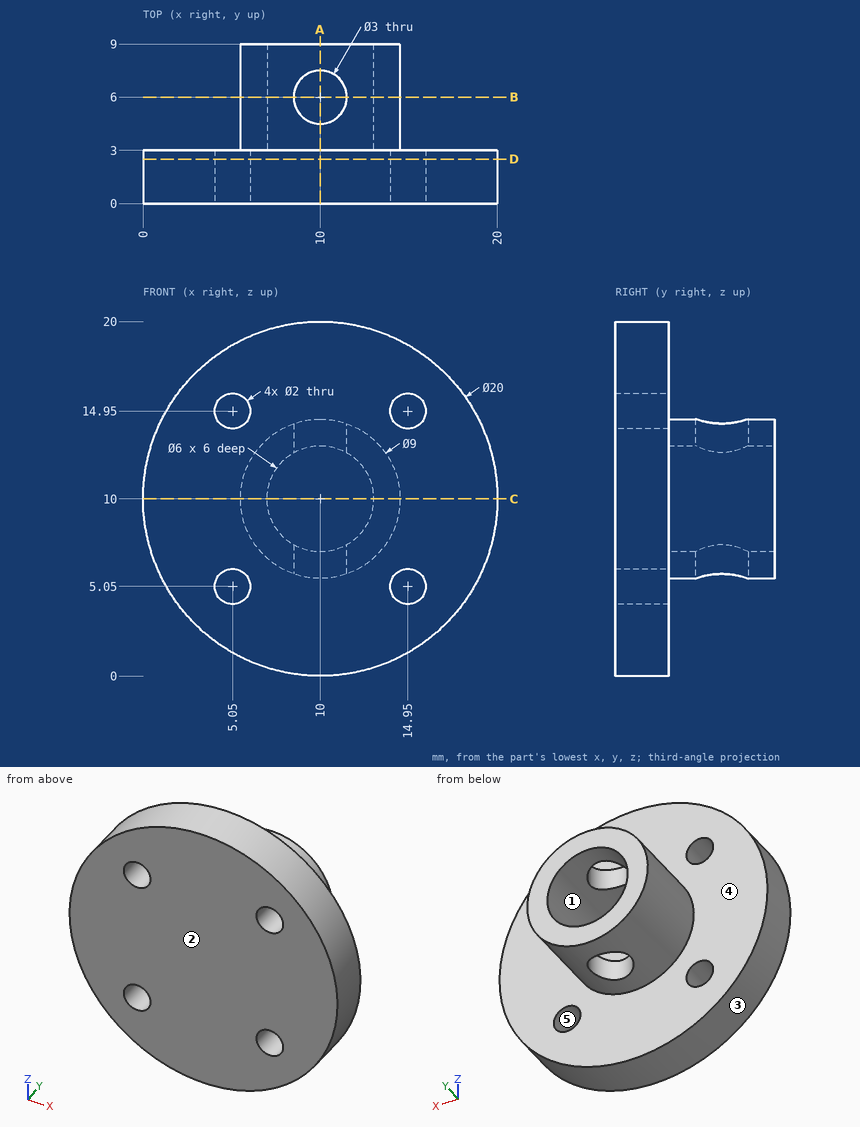
Answer from the drawing. Dimensions are ordinates in mm from the lowest x, y and z of the part. A direction names the side the tool comes from. Round coordinates to 2 decimals unless told otherwise and drop trailing zeros. Loops run counter-clockwise (first coordinate to the right, second up) from the corner with the lowest first, then second, coordinate; pieces in that order, holes last.
1) For the marked faces 1 and 2, determine the directions among +Z, -Z, +X, -X, +Y, -Y from which every point of the face is accessible in a straight line to the end or side of a thin tool.
Outcome:
face 1: +Y
face 2: +Z, -Z, +X, -X, -Y
2) Given P1, Ø5.5, axis at x = 10, z = 10, coming from the -Y side; P2, Ø4, axis at x = 10, y = 8, coming from the -Z side; P3, Ø2, axis at x = 15.5, y = 1.5, coming from the -Z side; P4, Ø1.5, axis at x = 12, y = 8, coming from the -Z side, each flat-ended and moving along its own axis, determine where each tip first touches the part or whether it passes through.
Outcome:
P1: stops at y = 0
P2: stops at z = 5.5
P3: stops at z = 1.07
P4: stops at z = 5.68
3) Consider line 1 (X direction, y = 5.25, z = 10); line 2 (Y direction, x = 5.5, z = 18); line 3 (Z direction, x = 15, y = 2.75). Determine where each line is inside the solid, lowest interval first.
Outcome:
line 1: x = 5.5 to 7, 13 to 14.5
line 2: y = 0 to 3
line 3: z = 1.34 to 4.05, 6.05 to 13.95, 15.95 to 18.66
4) For a pull along Z with two mould halves and no side action, classify the marked faces 3, 4 and 5 as released by +Z, released by -Z, zero draft, split by the parting line, or undercut.
Outcome:
face 3: split by the parting line
face 4: zero draft
face 5: undercut
5) A cutting plane is placed at C-C on z = 10. Determine the outline of the cut face in (x, y), plus the area to 3 significant figures.
Outcome:
outline: (0, 0) - (20, 0) - (20, 3) - (14.5, 3) - (14.5, 9) - (13, 9) - (13, 3) - (7, 3) - (7, 9) - (5.5, 9) - (5.5, 3) - (0, 3) - close
area: 78.0 mm2
6) A cutting plane is placed at B-B on y = 6. Determine the outline of the cut face in (x, z).
Outcome:
outline: (8.5, 5.76) - (8.5, 7.4) arc R3 cw to (8.5, 12.6) - (8.5, 14.24) arc R4.5 ccw to start; (11.5, 5.76) arc R4.5 ccw to (11.5, 14.24) - (11.5, 12.6) arc R3 cw to (11.5, 7.4) - close
7) A cutting plane is placed at D-D on y = 2.5. Determine the outline of the cut face in (x, z).
Outcome:
outline: circle Ø20 at (10, 10); hole circle Ø2 at (5.05, 5.05); hole circle Ø2 at (5.05, 14.95); hole circle Ø2 at (14.95, 5.05); hole circle Ø2 at (14.95, 14.95)
8) A cutting plane is placed at A-A on x = 10. Determine the outline of the cut face in (y, z).
Outcome:
outline: (0, 0) - (3, 0) - (3, 5.5) - (4.5, 5.5) - (4.5, 7) - (3, 7) - (3, 13) - (4.5, 13) - (4.5, 14.5) - (3, 14.5) - (3, 20) - (0, 20) - close; (7.5, 5.5) - (9, 5.5) - (9, 7) - (7.5, 7) - close; (7.5, 13) - (9, 13) - (9, 14.5) - (7.5, 14.5) - close
